from build123d import *

# Parameters (mm, degrees)
SKETCH1_W              = 453
SKETCH1_H              = 50
BASE_FLANGE1_DEPTH     = 3
SKETCHED_START         = -25
SKETCHED_BEND1_DEPTH   = 50
SKETCHED_BEND1_2_DEPTH = 50
SKETCH7_R              = 4
BOSS_EXTRUDE1_DEPTH    = 30


# Read off the part's stored shape, not the designer's step: Sketched Bend1
# Sheet-metal steps are written as plain solids
with BuildPart() as part:
    # Sketch1 → Base-Flange1 (new body)
    with BuildSketch(Plane.XY):
        Rectangle(SKETCH1_W, SKETCH1_H)
    extrude(amount=-BASE_FLANGE1_DEPTH)

    # Sketched Bend1 outline → Sketched Bend1 (cut)
    with BuildSketch(Plane(origin=(0, 0, 0), x_dir=(1, 0, 0), z_dir=(0, 1, 0)).offset(SKETCHED_START)):
        with BuildLine():
            ThreePointArc((-162.463865648, 2.795554958), (-161.69410853, 2.948669168), (-160.910951377, 3))
            Line((-160.910951377, 3), (-226.5, 3))
            Line((-226.5, 3), (-226.5, 0))
            Line((-226.5, 0), (-172.897018786, 0))
            Line((-172.897018786, 0), (-162.463865648, 2.795554958))
        make_face()
        with BuildLine():
            Line((226.5, 3), (160.910951377, 3))
            ThreePointArc((160.910951377, 3), (161.69410853, 2.948669168), (162.463865648, 2.795554958))
            Line((162.463865648, 2.795554958), (172.897018786, 0))
            Line((172.897018786, 0), (226.5, 0))
            Line((226.5, 0), (226.5, 3))
        make_face()
    extrude(amount=SKETCHED_BEND1_DEPTH, mode=Mode.SUBTRACT)

    # Sketched Bend1 2 outline → Sketched Bend1 2 (add)
    with BuildSketch(Plane(origin=(0, 0, 0), x_dir=(1, 0, 0), z_dir=(0, 1, 0)).offset(SKETCHED_START)):
        with BuildLine():
            Line((-160.910951377, 0), (-172.897018786, 0))
            Line((-172.897018786, 0), (-224.680067079, -13.875225972))
            Line((-224.680067079, -13.875225972), (-223.903609944, -16.773003451))
            Line((-223.903609944, -16.773003451), (-161.687408513, -0.102222521))
            ThreePointArc((-161.687408513, -0.102222521), (-161.302529954, -0.025665416), (-160.910951377, 0))
        make_face()
        with BuildLine():
            Line((224.680067079, -13.875225972), (172.897018786, 0))
            Line((172.897018786, 0), (160.910951377, 0))
            ThreePointArc((160.910951377, 0), (161.302529954, -0.025665416), (161.687408513, -0.102222521))
            Line((161.687408513, -0.102222521), (223.903609944, -16.773003451))
            Line((223.903609944, -16.773003451), (224.680067079, -13.875225972))
        make_face()
    extrude(amount=SKETCHED_BEND1_2_DEPTH)

    # Sketch7 → Boss-Extrude1 (add)
    with BuildSketch(Plane.XY):
        with Locations(Location((-100, 0, 0), (0, 0, 180))):
            Circle(SKETCH7_R)
        with Locations(Location((100, 0, 0), (0, 0, 180))):
            Circle(SKETCH7_R)
    extrude(amount=BOSS_EXTRUDE1_DEPTH)


solid = part.part
Design review of the part built by this model. Coordinates are the model's own, in mm. A direction names the side the tool comes from. Round coordinates to 2 decimals unless told otherwise and drop trailing zeros. Write each loop counter-clockwise with the first axis right and the second up, starting at its lowest first coordinate (ties: lowest second). Pieces come first, ordered by that corner, then holes. Notation, with made-up numbers: M -31,-4 L 24,-4 A32 ccw 24,23 Z; hole C 71.25,59.5 d5. An arc over 180 degrees is marked long. One line per item, written item: value. Start each with the question number.
1. Clearance check with flat-ended pins moving along their axes: P1, Ø12, axis at x = 155.5, y = -14.5, coming from the +Z side; P2, Ø25, axis at x = -42, y = -6.5, coming from the +Z side. State where each tip first meets the part, or that it passes through.
2. For faces 3 (the face through (-100, 0, 30)), 4 (the face through (192.36, -0.35, 8.32)), 5 (the face through (104, 0, 15)), list the 3-axis set-ups (+Z, -Z, +X, -X, +Y, -Y) from which the entire face can be reached by the end or side of a thin tool; tool diameter is ignored.
3. Take a section at D-D on x = -37. State the section outline as (y, z) points.
4. Take a section at C-C on x = 100. State the section outline as (y, z) points, then the cut area to 3 significant figures.
5. To check wall thickness, follow probe 1 along Z at (x, y) = (-86.5, -9.5); probe 2 along Z at (x, y) = (-205, -21); probe 3 along Y at (x, z) = (-99, 22.5). State the ranges of each line that lie inside material, in increasing order. Write a range as from..to.
6. Take a section at B-B on z = 4.5. State the section outline as (x, y) points.
7. Draft analysis for pull direction X (two halves, no side actions). For faces 1 (the face through (-1, -25, -0.5)), 2 (the face through (-2, 0, 0)), state which applies: pulls with the +X half, pulls with the -X half, needs draft (parallel to the pull), parting line crosses it, or undercut.
8. Take a section at A-A on y = 0. State the section outline as (x, z) points.
Computed:
1. P1: stops at z = 0.06
1. P2: stops at z = 0
2. face 3: +Z, +X, -X, +Y, -Y
2. face 4: +Z, +Y, -Y
2. face 5: +Z
3. outline: M -25,-3 L 25,-3 L 25,0 L -25,0 Z
4. outline: M -25,-3 L 25,-3 L 25,0 L 4,0 L 4,30 L -4,30 L -4,0 L -25,0 Z
4. area: 390 mm²
5. probe 1: z = -3..0
5. probe 2: z = 8.6..11.71
5. probe 3: y = -3.87..3.87
6. outline: M -189.69,-25 L -178.1,-25 L -178.1,25 L -189.69,25 Z; C -100,0 d8; C 100,0 d8; M 178.1,-25 L 189.69,-25 L 189.69,25 L 178.1,25 Z
7. face 1: needs draft
7. face 2: undercut
8. outline: M -224.68,13.88 L -162.46,-2.8 A6 ccw -160.91,-3 L 160.91,-3 A6 ccw 162.46,-2.8 L 224.68,13.88 L 223.9,16.77 L 161.69,0.1 A3 cw 160.91,0 L 104,0 L 104,30 L 96,30 L 96,0 L -96,0 L -96,30 L -104,30 L -104,0 L -160.91,0 A3 cw -161.69,0.1 L -223.9,16.77 Z
